Check sheet for the modelled part. Datum: model origin and axes. Units: mm. Face numbers are marked on the shaded views. Round coordinates to 2 decimals unless told otherwise and drop trailing zeros. Loops run counter-clockwise (first coordinate to the right, second up) from the corner with the lowest first, then second, coordinate; pieces in that order, holes last. Notation, with made-up numbers: (87, 55) - (132, 55) arc R35 cw to (132, 92) - close; hole circle Ø4 at (-35.5, 52.25). An arc over 180 degrees is marked (long way). Put each result on its own line as item: value. Start each with the question number.
Item 1: Section check D-D, the plane x = -40. Record the cut outline in (y, z), and give its area (3 significant figures).
Item 2: Section check A-A, the plane y = -10. Record the cut outline in (x, z), and give its area (3 significant figures).
Item 3: Gauge pin test, flat ends, axial feed: pin 1 Ø5 at (y, z) = (15, 4.5) entering from +X; pin 2 Ø4.5 at (x, z) = (-45, 2) entering from +Y; pin 3 Ø3 at (y, z) = (89, 2.5) entering from +X. Record the tip position at first contact, or that the pin passes through.
Item 4: Material ranges on line 1 along Y through (x, z) = (0, 0.65); line 2 along Y through (x, z) = (-45, 1.9); line 3 along Y through (x, z) = (0, 1.35), recorded low to high.
Item 5: Section check C-C, the plane z = 9.5. Record the cut outline in (x, y), and give its area (3 significant figures).
Item 6: Draft check along Y on the marked faces 1 and 2. Enter one of: pulls with the +Y half, pulls with the -Y half, needs draft (parallel to the pull), parting line crosses it, or undercut.
Item 7: Section check B-B, the plane x = 45. Record the cut outline in (y, z).
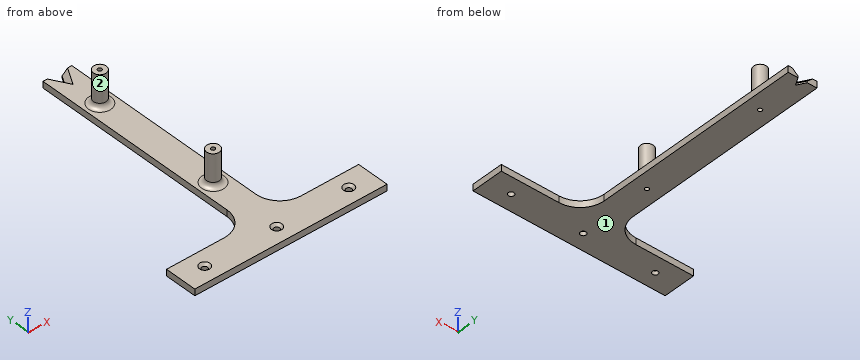
from build123d import *

# Parameters (mm, degrees)
SKETCH_R        = 1.75
SKETCH_R_2      = 1.25
PAD_DEPTH       = 4
SKETCH001_R     = 4
SKETCH001_R_2   = 1.25
PAD001_DEPTH    = 20
FILLET_R        = 3
FILLET001_R     = 3
CHAMFER_SIZE    = 1.5
CHAMFER001_SIZE = 3


with BuildPart() as part:
    # Sketch → Pad (new body)
    with BuildSketch(Plane.XY):
        with BuildLine():
            Line((-24, 0), (-60, 0))
            Line((-60, 0), (-60, -20))
            Line((-60, -20), (60, -20))
            Line((60, -20), (60, 0))
            Line((60, 0), (24, 0))
            ThreePointArc((9, 15), (13.393398, 4.393398), (24, 0))
            Line((9, 145), (9, 15))
            Line((2.886751, 145), (9, 145))
            Line((0, 140), (2.886751, 145))
            Line((-2.886751, 145), (0, 140))
            Line((-9, 145), (-2.886751, 145))
            Line((-9, 15), (-9, 145))
            ThreePointArc((-24, 0), (-13.393398, 4.393398), (-9, 15))
        make_face()
        with Locations((-45, -10)):
            Circle(SKETCH_R, mode=Mode.SUBTRACT)
        with Locations((45, -10)):
            Circle(SKETCH_R, mode=Mode.SUBTRACT)
        with Locations((0, -10)):
            Circle(SKETCH_R, mode=Mode.SUBTRACT)
        with Locations((0, 35)):
            Circle(SKETCH_R_2, mode=Mode.SUBTRACT)
        with Locations((0, 115)):
            Circle(SKETCH_R_2, mode=Mode.SUBTRACT)
    extrude(amount=PAD_DEPTH)

    # Sketch001 (on Face20 of Pad) → Pad001 (join)
    with BuildSketch(Plane.XY.offset(4)):
        with Locations((0, 115)):
            Circle(SKETCH001_R)
        with Locations((0, 115)):
            Circle(SKETCH001_R_2, mode=Mode.SUBTRACT)
        with Locations((0, 35)):
            Circle(SKETCH001_R)
        with Locations((0, 35)):
            Circle(SKETCH001_R_2, mode=Mode.SUBTRACT)
    extrude(amount=PAD001_DEPTH)

    # Fillet
    fillet_edges = [part.edges().sort_by_distance(p)[0] for p in [
        (-4, 115, 4),
    ]]
    fillet(fillet_edges, radius=FILLET_R)

    # Fillet001
    fillet001_edges = [part.edges().sort_by_distance(p)[0] for p in [
        (-4, 35, 4),
    ]]
    fillet(fillet001_edges, radius=FILLET001_R)

    # Chamfer
    chamfer_edges = [part.edges().sort_by_distance(p)[0] for p in [
        (43.25, -10, 4),
        (-1.75, -10, 4),
        (-46.75, -10, 4),
    ]]
    chamfer(chamfer_edges, length=CHAMFER_SIZE)

    # Chamfer001
    chamfer001_edges = [part.edges().sort_by_distance(p)[0] for p in [
        (1.443376, 142.5, 4),
        (-1.443376, 142.5, 4),
    ]]
    chamfer(chamfer001_edges, length=CHAMFER001_SIZE)


solid = part.part
Check result:
1. outline: (-20, 0) - (0, 0) - (0, 4) - (-20, 4) - close
1. area: 80.0 mm²
2. outline: (-60, 0) - (-46.75, 0) - (-46.75, 2.5) - (-48.25, 4) - (-60, 4) - close; (-43.25, 0) - (-1.75, 0) - (-1.75, 2.5) - (-3.25, 4) - (-41.75, 4) - (-43.25, 2.5) - close; (1.75, 0) - (43.25, 0) - (43.25, 2.5) - (41.75, 4) - (3.25, 4) - (1.75, 2.5) - close; (46.75, 0) - (60, 0) - (60, 4) - (48.25, 4) - (46.75, 2.5) - close
2. area: 431 mm²
3. pin 1: x = 9.2
3. pin 2: y = 0
3. pin 3: x = 9
4. line 1: -20 to -11.75, -8.25 to 33.75, 36.25 to 113.75, 116.25 to 140
4. line 2: -20 to -11.75, -8.25 to 0
4. line 3: -20 to -11.75, -8.25 to 33.75, 36.25 to 113.75, 116.25 to 139.3
5. outline: circle Ø8 at (0, 35); circle Ø8 at (0, 115); hole circle Ø2.5 at (0, 35); hole circle Ø2.5 at (0, 115)
5. area: 90.7 mm²
6. face 1: needs draft
6. face 2: undercut
7. outline: (-20, 0) - (-11.75, 0) - (-11.75, 2.5) - (-13.25, 4) - (-20, 4) - close; (-8.25, 0) - (0, 0) - (0, 4) - (-6.75, 4) - (-8.25, 2.5) - close
